Geometry: final body of the model. Coordinates: model frame, mm. Face numbers are marked on the shaded views. A direction names the side the tool comes from. Give positions to 0.01 mm unless a question says otherwise; leave off trailing zeros. Loops run counter-clockwise (first coordinate to the right, second up) from the corner with the lowest first, then second, coordinate; pieces in that order, holes last.
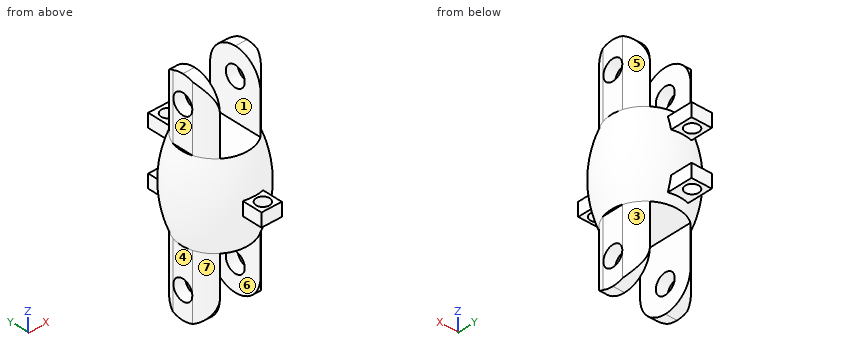
```python
from build123d import *

# Parameters (mm, degrees)
SKETCH3_W                = 19
SKETCH3_H                = 20
BOSS_EXTRUDE2_DEPTH      = 20
SKETCH4_W                = 19
SKETCH4_H                = 20
BOSS_EXTRUDE3_DEPTH      = 20
SKETCH5_R                = 15
SKETCH5_R_2              = 10
CUT_EXTRUDE1_DEPTH       = 49.347699066
SKETCH6_R                = 15
SKETCH6_R_2              = 10
CUT_EXTRUDE2_DEPTH       = 49.347699066
CUT_EXTRUDE3_DEPTH       = 37.996621535
CUT_EXTRUDE3_DEPTH_BACK  = 37.996621535
SKETCH7_W                = 12
SKETCH7_H                = 20
CUT_EXTRUDE4_DEPTH       = 40.430318363
CUT_EXTRUDE4_DEPTH_BACK  = 40.430318363
CUT_EXTRUDE5_DEPTH       = 40.430318445
CUT_EXTRUDE5_DEPTH_BACK  = 40.430318445
CUT_EXTRUDE8_DEPTH       = 42.188590816
CUT_EXTRUDE8_DEPTH_BACK  = 42.188590816
SKETCH10_R               = 3
SKETCH11_W               = 6
SKETCH11_H               = 4
BOSS_EXTRUDE5_DEPTH      = 18
SKETCH12_R               = 2
CUT_EXTRUDE9_DEPTH       = 41.871750794
SKETCH13_W               = 6
SKETCH13_H               = 4
BOSS_EXTRUDE6_DEPTH      = 18
CUT_EXTRUDE10_DEPTH      = 45.300113022
CUT_EXTRUDE10_DEPTH_BACK = 45.300113022
SKETCH14_R               = 2
SCALE1_SCALE             = 0.75


with BuildPart() as part:
    # Sketch2 → Revolve1 (revolve)
    with BuildSketch(Plane(origin=(0, 0, 0), x_dir=(0, 0, -1), z_dir=(1, 0, 0))):
        with BuildLine():
            Line((-12.5, 0), (12.5, 0))
            Line((12.5, 0), (12.5, 10))
            add(Edge.make_bspline(
                [(-12.5, 10), (0, 15), (12.5, 10)],
                knots=[0, 0, 0, 1, 1, 1], degree=2))
            Line((-12.5, 10), (-12.5, 0))
        make_face()
    revolve(axis=Axis((0, 0, 12.5), (0, 0, -1)))

    # Sketch3 → Boss-Extrude2 (add)
    with BuildSketch(Plane.XY.offset(12.5)):
        Rectangle(SKETCH3_W, SKETCH3_H)
    extrude(amount=BOSS_EXTRUDE2_DEPTH)

    # Sketch4 → Boss-Extrude3 (add)
    with BuildSketch(Plane(origin=(0, 0, -12.5), x_dir=(-1, 0, 0), z_dir=(0, 0, -1))):
        Rectangle(SKETCH4_W, SKETCH4_H)
    extrude(amount=BOSS_EXTRUDE3_DEPTH)

    # Sketch5 → Cut-Extrude1 (cut, through all)
    with BuildSketch(Plane(origin=(0, 0, -12.5), x_dir=(-1, 0, 0), z_dir=(0, 0, -1))):
        Circle(SKETCH5_R)
        Circle(SKETCH5_R_2, mode=Mode.SUBTRACT)
    extrude(amount=CUT_EXTRUDE1_DEPTH, mode=Mode.SUBTRACT)

    # Sketch6 → Cut-Extrude2 (cut, through all)
    with BuildSketch(Plane.XY.offset(12.5)):
        Circle(SKETCH6_R)
        Circle(SKETCH6_R_2, mode=Mode.SUBTRACT)
    extrude(amount=CUT_EXTRUDE2_DEPTH, mode=Mode.SUBTRACT)

    # Sketch7 → Cut-Extrude3 (cut, two sides: drawn at the far end of the back side and taken through both)
    with BuildSketch(Plane(origin=(0, 0, 0), x_dir=(1, 0, 0), z_dir=(0, 1, 0)).offset(-CUT_EXTRUDE3_DEPTH_BACK)):
        with Locations((0, 22.5)):
            Rectangle(SKETCH7_W, SKETCH7_H)
        with Locations((0, -22.5)):
            Rectangle(SKETCH7_W, SKETCH7_H)
    extrude(amount=CUT_EXTRUDE3_DEPTH + CUT_EXTRUDE3_DEPTH_BACK, mode=Mode.SUBTRACT)

    # Sketch8 → Cut-Extrude4 (cut, two sides: drawn at the far end of the back side and taken through both)
    with BuildSketch(Plane(origin=(-6, 0, 0), x_dir=(0, 0, -1), z_dir=(1, 0, 0)).offset(-CUT_EXTRUDE4_DEPTH_BACK)):
        with BuildLine():
            Line((-32.5, 8), (-32.5, -5.1e-08))
            ThreePointArc((-32.5, -5.1e-08), (-30.156854267, 5.656854232), (-24.5, 8))
            Line((-24.5, 8), (-32.5, 8))
        make_face()
        with BuildLine():
            Line((-32.5, -8), (-24.5, -8))
            ThreePointArc((-24.5, -8), (-30.156854232, -5.656854267), (-32.5, -5.1e-08))
            Line((-32.5, -5.1e-08), (-32.5, -8))
        make_face()
    extrude(amount=CUT_EXTRUDE4_DEPTH + CUT_EXTRUDE4_DEPTH_BACK, mode=Mode.SUBTRACT)

    # Sketch9 → Cut-Extrude5 (cut, two sides: drawn at the far end of the back side and taken through both)
    with BuildSketch(Plane(origin=(-6, 0, 0), x_dir=(0, 0, -1), z_dir=(1, 0, 0)).offset(-CUT_EXTRUDE5_DEPTH_BACK)):
        with BuildLine():
            ThreePointArc((24.5, 8), (30.156854249, 5.656854249), (32.5, 0))
            Line((32.5, 0), (32.5, 8))
            Line((32.5, 8), (24.5, 8))
        make_face()
        with BuildLine():
            ThreePointArc((32.5, 0), (30.156854249, -5.656854249), (24.5, -8))
            Line((24.5, -8), (32.5, -8))
            Line((32.5, -8), (32.5, 0))
        make_face()
    extrude(amount=CUT_EXTRUDE5_DEPTH + CUT_EXTRUDE5_DEPTH_BACK, mode=Mode.SUBTRACT)

    # Sketch10 → Cut-Extrude8 (cut, two sides: drawn at the far end of the back side and taken through both)
    with BuildSketch(Plane(origin=(9.5, 0, 0), x_dir=(0, 0, -1), z_dir=(1, 0, 0)).offset(-CUT_EXTRUDE8_DEPTH_BACK)):
        with Locations((24.5, 0)):
            Circle(SKETCH10_R)
        with Locations((-24.5, 0)):
            Circle(SKETCH10_R)
    extrude(amount=CUT_EXTRUDE8_DEPTH + CUT_EXTRUDE8_DEPTH_BACK, mode=Mode.SUBTRACT)

    # Sketch11 → Boss-Extrude5 (add)
    with BuildSketch(Plane(origin=(0, 0, 0), x_dir=(1, 0, 0), z_dir=(0, 1, 0))):
        Rectangle(SKETCH11_W, SKETCH11_H)
    extrude(amount=-BOSS_EXTRUDE5_DEPTH)

    # Sketch12 → Cut-Extrude9 (cut, through all)
    with BuildSketch(Plane(origin=(0, 0, -2), x_dir=(-1, 0, 0), z_dir=(0, 0, -1))):
        with Locations((0, -15.218)):
            Circle(SKETCH12_R)
    extrude(amount=-CUT_EXTRUDE9_DEPTH, mode=Mode.SUBTRACT)

    # Sketch13 → Boss-Extrude6 (add)
    with BuildSketch(Plane(origin=(0, 0, 0), x_dir=(1, 0, 0), z_dir=(0, 1, 0))):
        with Locations((0, 8)):
            Rectangle(SKETCH13_W, SKETCH13_H)
        with Locations((0, -8)):
            Rectangle(SKETCH13_W, SKETCH13_H)
    extrude(amount=BOSS_EXTRUDE6_DEPTH)

    # Sketch14 → Cut-Extrude10 (cut, two sides: drawn at the far end of the back side and taken through both)
    with BuildSketch(Plane.XY.offset(-6).offset(-CUT_EXTRUDE10_DEPTH_BACK)):
        with Locations((0, 14.962)):
            Circle(SKETCH14_R)
    extrude(amount=CUT_EXTRUDE10_DEPTH + CUT_EXTRUDE10_DEPTH_BACK, mode=Mode.SUBTRACT)


with BuildPart() as part_1:
    # Scale1: scaled about (2.6e-08, 0.137076755, -6.1e-08)
    add(part.part.scale(SCALE1_SCALE).moved(Location((7e-09, 0.034269189, -1.5e-08))))


solid = part_1.part
```
Q1. Material intervals for probe 1 along Z at (x, y) = (1.5, 2) (3 decimals); probe 2 along Y at (x, z) = (0, -6.7); probe 3 along X at (y, z) = (-4.25, 20), sorted ascending.
Q2. Section query A-A, the plane z = -12.5. Return loops of the section in (x, y) (3 decimals), and give its area (3 significant figures).
Q3. Mould query, pull axis X, two halves, no side actions, for the marked faces 1, 2 and 3. Classes: +X half, -X half, draft (parallel to the pull), parting line (faces both ways), or undercut.
Q4. Section query B-B, the plane y = 1. State how many separate pieces and enclosed holes the cut face has, and give its area (3 significant figures).
Q5. Reachability of the marked faces 4, 5, 6 and 7 from +Z, -Z, +X, -X, +Y, -Y: full face, straight path, thin tool, end or side. Return the list, or none.
Q6. Pin query (flat end, axial travel): pin 1 Ø3.5 at (y, z) = (-1, 20) entering from -X (3 decimals); pin 2 Ø3.5 at (y, z) = (-1.5, -16.5) entering from +X (3 decimals); pin 3 Ø4 at (x, y) = (-1, -7.5) entering from +Z (3 decimals); pin 4 Ø4 at (y, z) = (0.03, -18.38) entering from +X. Return the tip coordinate at first contact, or that it passes through.
Resolved:
1. probe 1: z = -9.375 to 9.375
1. probe 2: y = -8.38 to 9.76, 12.76 to 13.53
1. probe 3: x = -6.16 to -4.5, 4.5 to 6.16
2. outline: (-7.125, -2.308) arc R7.5 ccw to (-4.5, -5.966) - (-4.5, 6.034) arc R7.5 ccw to (-7.125, 2.376) - close; (4.5, -5.966) arc R7.5 ccw to (7.125, -2.308) - (7.125, 2.376) arc R7.5 ccw to (4.5, 6.034) - close
2. area: 48.0 mm2
3. face 1: undercut
3. face 2: -X half
3. face 3: +X half
4. separate pieces: 5
4. enclosed holes: 0
4. area: 440 mm2
5. face 4: -Z, -X, +Y, -Y
5. face 5: +Z, +X, +Y
5. face 6: -Z, +Y, -Y
5. face 7: -Z, -X, -Y
6. pin 1: stops at x = -7.125
6. pin 2: stops at x = 7.125
6. pin 3: stops at z = 9.375
6. pin 4: passes through
